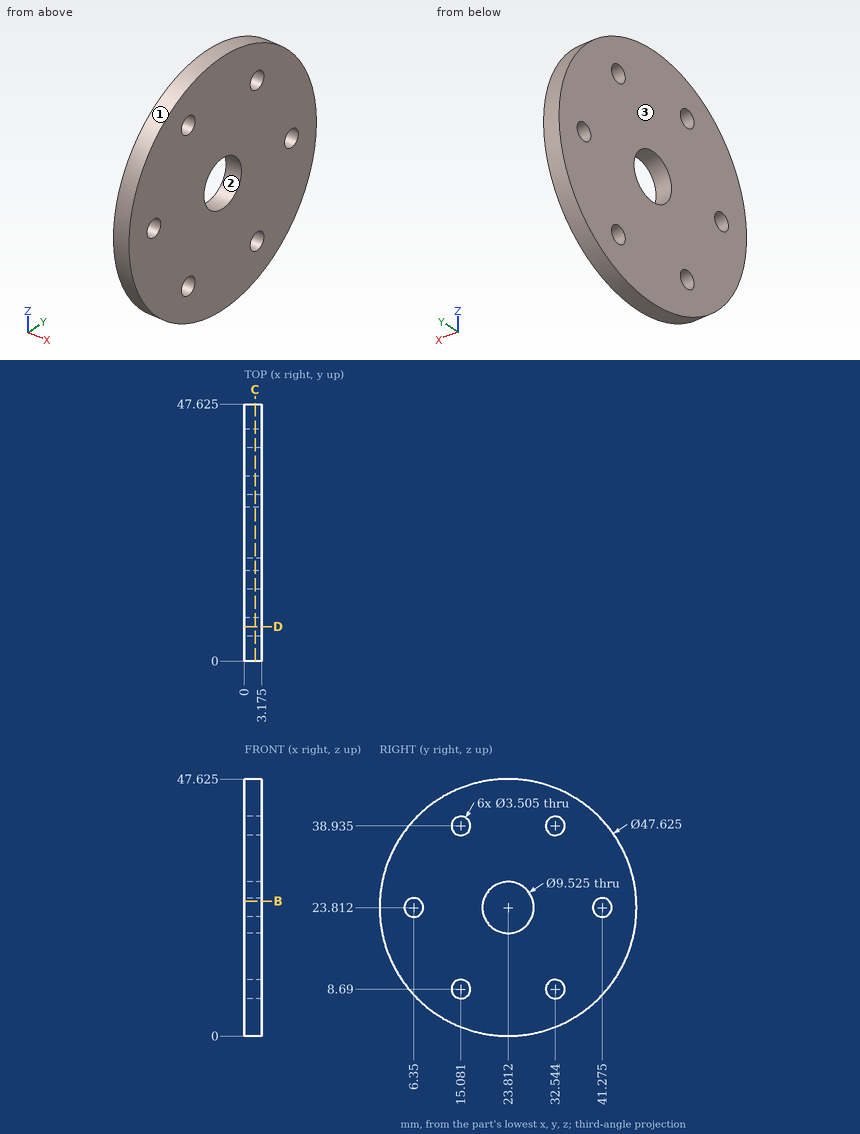
The figure shows three views and two pictorial views of one solid part (mm, origin at its lowest corner). Answer the questions. Round coordinates to 2 decimals unless told otherwise and drop trailing zeros. Loops run counter-clockwise (first coordinate to the right, second up) from the corner with the lowest first, then second, coordinate; pieces in that order, holes last. Notation, with made-up numbers: (-9.5, 80) - (7.5, 80) arc R17 cw to (7.5, 100) - close; hole circle Ø11 at (89.5, 57). An arc over 180 degrees is marked (long way). Use one line per item in the form item = value. Start each with the question number.
(1) Find section C-C on x = 2. Give the number of separate pieces and of enclosed holes in the cut face, and give its area (3 significant figures).
(2) A flat-ended cylindrical pin translates along its axis: P1, Ø1, axis at x = 0.5, z = 38, coming from the -Y side. Find the tip coordinate at first contact, or state that the pin passes through.
(3) Consider line 1 (Y direction, x = 0.3, z = 8) (1 decimal); line 2 (Y direction, x = 1.45, z = 7.5) (1 decimal); line 3 (Y direction, x = 2.05, z = 23) (1 decimal). Determine where each line is inside the solid, lowest interval first.
(4) Find section B-B on z = 25. Determine the outline of the cut face in (x, y) (1 decimal).
(5) Determine the mould class of the marked faces 1, 2 and 3 for opening direction Y: +Y half, -Y half, draft (parallel to the pull), parting line (faces both ways), or undercut.
(6) Find section D-D on y = 6.35. Determine the outline of the cut face in (x, z) (1 decimal).
Answer list:
q1.separate_pieces = 1
q1.enclosed_holes = 7
q1.area = 1,650 mm^2
q2.P1 = 4.33
q3.line_1 = 6 to 13.5, 16.7 to 30.9, 34.2 to 41.6
q3.line_2 = 6.5 to 13.8, 16.4 to 31.3, 33.8 to 41.2
q3.line_3 = 0 to 4.8, 7.9 to 19.1, 28.5 to 39.7, 42.8 to 47.6
q4.outline = (0, 0) - (3.2, 0) - (3.2, 5.1) - (0, 5.1) - close; (0, 7.6) - (3.2, 7.6) - (3.2, 19.2) - (0, 19.2) - close; (0, 28.4) - (3.2, 28.4) - (3.2, 40) - (0, 40) - close; (0, 42.6) - (3.2, 42.6) - (3.2, 47.6) - (0, 47.6) - close
q5.face_1 = parting line
q5.face_2 = undercut
q5.face_3 = draft
q6.outline = (0, 7.6) - (3.2, 7.6) - (3.2, 22.1) - (0, 22.1) - close; (0, 25.6) - (3.2, 25.6) - (3.2, 40) - (0, 40) - close
